Read the model definition and answer for the solid it produces. Units are mm, in the model's axes. Coordinates: 2 decimals unless noted, no trailing zeros. Order: outer loops, then holes, each group sorted by start corner. A loop starts at its lowest first (then second) coordinate and runs counter-clockwise, first axis right, second up. Notation, with made-up numbers: (-9.5, 66) -> (48.5, 66) arc R12 cw to (48.5, 71) -> close; hole circle Ø7 at (-32, 16). An arc over 180 degrees is marked (long way). Answer as a JSON object with one key per item and string values. Group by question number.
1) Section C-C on z = 11 is taken. Determine the outline of the cut face in (x, y).
2) Given pin 1 (0.6 mm diameter, centred on y = 0.5, z = 29.5, fed in from -X), flat-ended and moving along its own axis, determine where the tip first touches the part or whether it passes through.
3) Consider L1, parallel to X at y = 1.1, z = 28.5; L2, parallel to Z at x = -16.5, y = 0.9; L3, parallel to X at y = 0.8, z = 19. Determine where each line is inside the solid, lowest interval first.
4) Section A-A on y = 1.2 is taken. Count the separate pieces of the cut face and the enclosed holes in it, and give its area (3 significant figures).
5) Section B-B on x = -21 is taken. Determine the outline of the cut face in (y, z), and give its area (3 significant figures).
from build123d import *

# Parameters (mm, degrees)
SKETCH_1_R      = 0.75
EXTRUDE_2_DEPTH = 1.5


with BuildPart() as part:
    # 草图1 → 凸台-拉伸2 (new body)
    with BuildSketch(Plane(origin=(0, 0, 0), x_dir=(1, 0, 0), z_dir=(0, 1, 0))):
        with BuildLine():
            Line((28.831406487, -10), (30, -10))
            ThreePointArc((30, -10), (33.535533906, -8.535533906), (35, -5))
            Line((35, -5), (35, 0))
            Line((35, 0), (35, 5))
            ThreePointArc((35, 5), (33.535533906, 8.535533906), (30, 10))
            Line((30, 10), (28.831406487, 10))
            ThreePointArc((28.831406487, 10), (26.237033878, 10.725747929), (24.395805489, 12.692307692))
            ThreePointArc((24.395805489, 12.692307692), (19.445436483, 19.445436483), (12.692307692, 24.395805489))
            ThreePointArc((12.692307692, 24.395805489), (10.725747929, 26.237033878), (10, 28.831406487))
            Line((10, 28.831406487), (10, 30))
            ThreePointArc((10, 30), (8.535533906, 33.535533906), (5, 35))
            Line((5, 35), (0, 35))
            Line((0, 35), (-5, 35))
            ThreePointArc((-5, 35), (-8.535533906, 33.535533906), (-10, 30))
            Line((-10, 30), (-10, 28.831406487))
            ThreePointArc((-10, 28.831406487), (-10.725747929, 26.237033878), (-12.692307692, 24.395805489))
            ThreePointArc((-12.692307692, 24.395805489), (-19.445436483, 19.445436483), (-24.395805489, 12.692307692))
            ThreePointArc((-24.395805489, 12.692307692), (-26.237033878, 10.725747929), (-28.831406487, 10))
            Line((-28.831406487, 10), (-30, 10))
            ThreePointArc((-30, 10), (-33.535533906, 8.535533906), (-35, 5))
            Line((-35, 5), (-35, 0))
            Line((-35, 0), (-35, -5))
            ThreePointArc((-35, -5), (-33.535533906, -8.535533906), (-30, -10))
            Line((-30, -10), (-28.831406487, -10))
            ThreePointArc((-28.831406487, -10), (-26.237033878, -10.725747929), (-24.395805489, -12.692307692))
            ThreePointArc((-24.395805489, -12.692307692), (-19.445436483, -19.445436483), (-12.692307692, -24.395805489))
            ThreePointArc((-12.692307692, -24.395805489), (-10.725747929, -26.237033878), (-10, -28.831406487))
            Line((-10, -28.831406487), (-10, -30))
            ThreePointArc((-10, -30), (-8.535533906, -33.535533906), (-5, -35))
            Line((-5, -35), (0, -35))
            Line((0, -35), (5, -35))
            ThreePointArc((5, -35), (8.535533906, -33.535533906), (10, -30))
            Line((10, -30), (10, -28.831406487))
            ThreePointArc((10, -28.831406487), (10.725747929, -26.237033878), (12.692307692, -24.395805489))
            ThreePointArc((12.692307692, -24.395805489), (19.445436483, -19.445436483), (24.395805489, -12.692307692))
            ThreePointArc((24.395805489, -12.692307692), (26.237033878, -10.725747929), (28.831406487, -10))
        make_face()
        with Locations(Location((15.909902577, -15.909902577, 0), (0, 0, 270))):
            Circle(SKETCH_1_R, mode=Mode.SUBTRACT)
        with Locations(Location((-15.909902577, -15.909902577, 0), (0, 0, 270))):
            Circle(SKETCH_1_R, mode=Mode.SUBTRACT)
        with Locations(Location((-15.909902577, 15.909902577, 0), (0, 0, 270))):
            Circle(SKETCH_1_R, mode=Mode.SUBTRACT)
        with Locations(Location((15.909902577, 15.909902577, 0), (0, 0, 270))):
            Circle(SKETCH_1_R, mode=Mode.SUBTRACT)
    extrude(amount=EXTRUDE_2_DEPTH)


solid = part.part
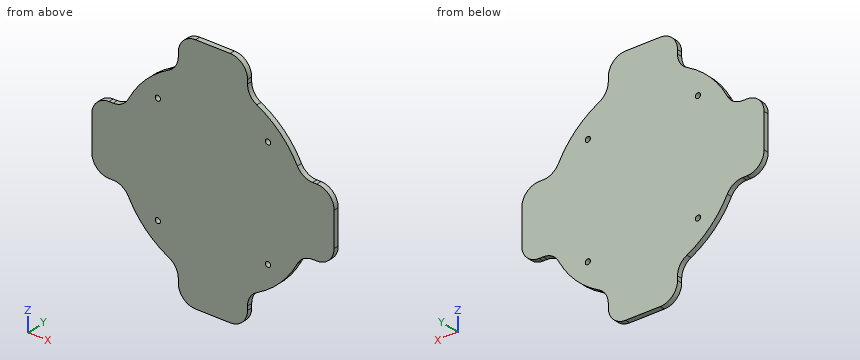
Worked answers:
{
 "1": {"outline": "(-25.83, 0) -> (25.83, 0) -> (25.83, 1.5) -> (-25.83, 1.5) -> close"},
 "2": {"pin 1": "stops at x = -10"},
 "3": {"L1": "x = -10.01 to 10.01", "L2": "z = -22 to -16.37, -15.45 to 15.45, 16.37 to 22", "L3": "x = -19.88 to 19.88"},
 "4": {"separate pieces": "1", "enclosed holes": "4", "area": "2,990 mm²"},
 "5": {"outline": "(0, -17.76) -> (1.5, -17.76) -> (1.5, 17.76) -> (0, 17.76) -> close", "area": "53.3 mm²"}
}
